Model file for the job. Use its own axes, mm. A direction names the side the tool comes from. Give positions to 0.01 mm unless a question says otherwise; leave off trailing zeros. Write each loop counter-clockwise with the first axis right and the second up, starting at its lowest first coordinate (ties: lowest second). Pieces come first, ordered by that corner, then holes. Notation, with made-up numbers: M 61,31 L 112,31 A17 ccw 112,63 Z; hole C 89.5,17 d10. An arc over 180 degrees is marked long. Answer as a JSON object with one key per item and string values. Group by question number.
```python
from build123d import *

# Parameters (mm, degrees)
SALIENTE_EXTRUIR1_DEPTH = 100
SKETCH3_W               = 10.723679857
SKETCH3_H               = 38.227553418
CUT_EXTRUDE1_DEPTH      = 27
SKETCH5_R               = 19.056213919
CUT_EXTRUDE2_DEPTH      = 4.078011603
CUT_EXTRUDE3_DEPTH      = 8
SKETCH7_W               = 15.237542525
SKETCH7_H               = 35.999775061
CUT_EXTRUDE4_DEPTH      = 5.8
FILLET1_R               = 10
FILLET2_R               = 10
FILLET3_R               = 5
SKETCH8_W               = 14.627019037
SKETCH8_H               = 6.752783555
BOSS_EXTRUDE1_DEPTH     = 2
SKETCH11_W              = 54
SKETCH11_H              = 35
CUT_EXTRUDE6_DEPTH      = 19
SKETCH12_W              = 5.502183779
SKETCH12_H              = 5.157792635
CUT_EXTRUDE7_DEPTH      = 9
BOSS_EXTRUDE2_START     = 8
BOSS_EXTRUDE2_DEPTH     = 8
FILLET4_R               = 2
FILLET5_R               = 2


with BuildPart() as part:
    # Croquis1 → Saliente-Extruir1 (new body)
    with BuildSketch(Plane(origin=(0, 0, 0), x_dir=(1, 0, 0), z_dir=(0, 1, 0))):
        Polygon((-22.831092882, -9.100137773), (-21.539334245, -9.100137773), (-21.539334245, -6.453403554), (-25.857066178, -6.453403554), (-25.857066178, 0), (28.142933822, 0), (28.142933822, -6.453403554), (23.825201889, -6.453403554), (23.825201889, -9.100137773), (25.116960526, -9.100137773), (22.625201889, -11.232188763), (20.133443253, -9.100137773), (21.425201889, -9.100137773), (21.425201889, -6.453403554), (-19.139334245, -6.453403554), (-19.139334245, -9.100137773), (-17.847575609, -9.100137773), (-20.339334245, -11.232188763), align=None)
    extrude(amount=SALIENTE_EXTRUIR1_DEPTH)

    # Sketch3 → Cut-Extrude1 (cut)
    with BuildSketch(Plane.ZY.offset(25.857066178)):
        with Locations((7.73723188, 67.748563888)):
            Rectangle(SKETCH3_W, SKETCH3_H)
    extrude(amount=-CUT_EXTRUDE1_DEPTH, mode=Mode.SUBTRACT)

    # Sketch5 → Cut-Extrude2 (cut)
    with BuildSketch(Plane.XY.offset(6.453403554)):
        with Locations((1.142933822, 68.165450094)):
            Circle(SKETCH5_R)
    extrude(amount=-CUT_EXTRUDE2_DEPTH, mode=Mode.SUBTRACT)

    # Sketch6 → Cut-Extrude3 (cut)
    with BuildSketch(Plane(origin=(0, 0, 0), x_dir=(-1, 0, 0), z_dir=(0, 0, -1))):
        with BuildLine():
            ThreePointArc((-28.142933822, 100), (-1.142933822, 91.515299145), (25.857066178, 100))
            ThreePointArc((25.857066178, 100), (-1.142933822, 109.141720496), (-28.142933822, 100))
        make_face()
    extrude(amount=-CUT_EXTRUDE3_DEPTH, mode=Mode.SUBTRACT)

    # Sketch7 → Cut-Extrude4 (cut)
    with BuildSketch(Plane(origin=(0, 0, 0), x_dir=(-1, 0, 0), z_dir=(0, 0, -1))):
        with Locations((18.238294915, 66.88524583)):
            Rectangle(SKETCH7_W, SKETCH7_H)
    extrude(amount=-CUT_EXTRUDE4_DEPTH, mode=Mode.SUBTRACT)

    # Fillet1
    fillet1_edges = [part.edges().sort_by_distance(p)[0] for p in [
        (-25.857066178, 84.885133361, 1.187695976),
    ]]
    fillet(fillet1_edges, radius=FILLET1_R)

    # Fillet2
    fillet2_edges = [part.edges().sort_by_distance(p)[0] for p in [
        (-10.619523653, 48.8853583, 1.187695976),
    ]]
    fillet(fillet2_edges, radius=FILLET2_R)

    # Fillet3
    fillet3_edges = [part.edges().sort_by_distance(p)[0] for p in [
        (-10.619523653, 84.885133361, 1.187695976),
    ]]
    fillet(fillet3_edges, radius=FILLET3_R)

    # Sketch8 → Boss-Extrude1 (add)
    with BuildSketch(Plane(origin=(28.142933822, 0, 0), x_dir=(0, 0, -1), z_dir=(1, 0, 0))):
        with Locations((-7.313509519, 96.623608222)):
            Rectangle(SKETCH8_W, SKETCH8_H)
    extrude(amount=BOSS_EXTRUDE1_DEPTH)

    # Sketch11 → Cut-Extrude6 (cut)
    with BuildSketch(Plane(origin=(0, 0, 0), x_dir=(-1, 0, 0), z_dir=(0, 0, -1))):
        with Locations((-1.142933822, 17.5)):
            Rectangle(SKETCH11_W, SKETCH11_H)
    extrude(amount=-CUT_EXTRUDE6_DEPTH, mode=Mode.SUBTRACT)

    # Sketch12 → Cut-Extrude7 (cut)
    with BuildSketch(Plane.XZ.offset(-86.862340597)):
        with Locations((-20.48547756, 9.032299872)):
            Rectangle(SKETCH12_W, SKETCH12_H)
    extrude(amount=-CUT_EXTRUDE7_DEPTH, mode=Mode.SUBTRACT)

    # Sketch13 → Boss-Extrude2 (add)
    with BuildSketch(Plane(origin=(0, 0, 8), x_dir=(-1, 0, 0), z_dir=(0, 0, -1)).offset(BOSS_EXTRUDE2_START)):
        with BuildLine():
            Line((21.539334245, 100), (19.139334245, 100))
            Line((19.139334245, 100), (19.139334245, 96.095020365))
            ThreePointArc((19.139334245, 96.095020365), (20.348097119, 96.6915372), (21.539334245, 97.322325698))
            Line((21.539334245, 97.322325698), (21.539334245, 100))
        make_face()
    extrude(amount=-BOSS_EXTRUDE2_DEPTH)

    # Fillet4
    # the kernel refuses this fillet: 2 mm, written as the material it adds along each edge
    with BuildSketch(Plane(origin=(-21.539334245, 97.322325698, 0), x_dir=(0, 1, 0), z_dir=(0, 0, 1))) as fillet4_piece_1:
        with BuildLine():
            CenterArc((3.431070837, 1.852672033), FILLET4_R, 147.126635273, 100.744049636)
            Line((1.751326275, 2.938240182), (1.717731384, 2.959951545))
            ThreePointArc((1.717731384, 2.959951545), (0.814679242, 1.505469297), (-0.035079002, 0.019221436))
            Line((-0.035079002, 0.019221436), (0, -0.04))
            ThreePointArc((0, -0.04), (1.338837151, -0.04), (2.662606371, -0.037053441))
            Line((2.662606371, -0.037053441), (2.677674302, 0))
        make_face()
    extrude(amount=6.453403554)

    # Fillet5
    fillet5_edges = [part.edges().sort_by_distance(p)[0] for p in [
        (-19.139334245, 96.095020365, 3.226701777),
    ]]
    fillet(fillet5_edges, radius=FILLET5_R)


solid = part.part
```
Q1. Slice it at D-D, the plane z = 4.5. Write the cut outline in (x, y).
Q2. Wall check: L1, parallel to X at y = 96, z = 9; L2, parallel to Z at x = -6, y = 65.5; L3, parallel to Z at x = 14, y = 51. Give the ranges that are in metal, low to high.
Q3. 3-axis set-ups, long thin cutter, end or side, ignore diameter. For faces 5 (the cylindrical face through (-25.162, 99.524, 3.182)), 6 (the cylindrical face through (-22.81, 98.84, 3.18)), 7 (the flat face through (-12, 86.862, 4)), 8 (the flat face through (-23, 48.885, 1)): which of +Z, -Z, +X, -X, +Y, -Y reach the whole face in a straight line?
Q4. Two-plate mould, pull along Y, no slides. Class faces 1 (the flat face through (21.425, 67, 8)), 2 (the flat face through (2, 35, 3)), 3 (the flat face through (23, 100, 9)), 4 (the flat face through (-13, 48.635, 5)): +Y half, -Y half, draft (parallel to the pull), parting line (faces both ways), or undercut.
Q5. Slice it at B-B, the plane y = 43. Write the cut outline in (x, z), then the cut area to 3 significant figures.
Q6. Drop flat-ended pins along their axis: P1, Ø3, axis at y = 75.5, z = 12, coming from the -X side; P2, Ø3, axis at y = 54, z = 4.5, coming from the +X side; P3, Ø1, axis at x = -10, y = 90.5, coming from the +Z side. Give the stop position or say it passes through.
Q7. Slice it at C-C, the plane x = 9. Write the cut outline in (y, z).
Q8. Slice it at A-A, the plane z = 10. Write the cut outline in (x, y).
Solved:
{
 "1": {"outline": "M -25.86,35 L 28.14,35 L 28.14,93.25 L 30.14,93.25 L 30.14,100 L 28.14,100 A47.2 cw -17.95,95.55 A2 cw -19.14,97.38 L -19.14,100 L -21.54,100 A2 cw -24.48,99.07 A47.2 cw -25.86,100 L -25.86,94.89 A10 ccw -21.83,86.86 L -2.54,86.86 A19.06 cw long 1.14,49.11 L 1.14,48.63 L -25.86,48.63 Z"},
 "2": {"L1": "x = -21.54 to -19.14, 21.43 to 23.83, 28.14 to 30.14", "L2": "z = 0 to 2.38", "L3": "z = 0 to 6.45"},
 "3": {"face 5": "+Z, -Z, +Y", "face 6": "-Z, +Y", "face 7": "+Z, -X", "face 8": "+Z, -Z, -X"},
 "4": {"face 1": "draft", "face 2": "-Y half", "face 3": "+Y half", "face 4": "undercut"},
 "5": {"outline": "M -25.86,0 L 28.14,0 L 28.14,6.45 L 23.83,6.45 L 23.83,9.1 L 25.12,9.1 L 22.63,11.23 L 20.13,9.1 L 21.43,9.1 L 21.43,6.45 L -19.14,6.45 L -19.14,9.1 L -17.85,9.1 L -20.34,11.23 L -22.83,9.1 L -21.54,9.1 L -21.54,6.45 L -25.86,6.45 Z", "area": "372 mm²"},
 "6": {"P1": "stops at x = 21.77", "P2": "stops at x = 28.14", "P3": "stops at z = 6.45"},
 "7": {"outline": "M 35,0 L 92.17,0 L 92.17,6.45 L 85.53,6.45 L 85.53,2.38 L 50.8,2.38 L 50.8,6.45 L 35,6.45 Z"},
 "8": {"outline": "M -21.78,35 L -18.9,35 L -18.9,48.63 L -21.78,48.63 Z; M -21.78,95.86 L -18.9,95.86 L -18.9,100 L -21.78,100 Z; M 21.19,35 L 24.07,35 L 24.07,100 L 21.19,100 Z; M 28.14,93.25 L 30.14,93.25 L 30.14,100 L 28.14,100 Z"}
}
